```python
from build123d import *

# Parameters (mm, degrees)
F1_DEPTH     = 7.5
F2_R         = 1.5
F3_R         = 1.5
F4_F1_R      = 1
F4_F2_R      = 1
F5_W         = 10
F5_H         = 10
F6_DEPTH     = 1
F7_T1_DEPTH  = 5
F7_T3_DEPTH  = 7.5
F7_T9_DEPTH  = 11.0917464655
F7_T14_DEPTH = 15
F7_T22_DEPTH = 15
F7_T27_DEPTH = 11.0917464655


# Not quite as in the source:
# - a fillet or chamfer that OpenCascade refuses, or shapes differently, is made with other operations: its cross-section is extruded or revolved along the edge and cut away or added


with BuildPart() as f1:
    # F0 (on Front) → F1 (new body)
    with BuildSketch(Plane.XZ):
        Polygon((0, 0), (0, 5), (-14.5909318536, 5), (-495, 5), (-500, 5), (-500, 0), (-500, -195), (-495, -195), (-408.1860127931, -160.8005504943), align=None)
        Polygon((-26.1103633187, -4.911916504), (-410.018635385, -156.1485085302), (-495, -189.6260158027), (-495, -142.4539996661), (-495, -95.2819835295), (-495, -93.9333955313), (-494.06737982, -93.7563320577), align=None, mode=Mode.SUBTRACT)
        Polygon((-495, 0), (-27.044750547, 0), (-495, -88.8440800691), (-495, -44.4220400346), align=None, mode=Mode.SUBTRACT)
    extrude(amount=F1_DEPTH)

    # F2
    f2_edges = [f1.edges().sort_by_distance(p)[0] for p in [
        (-495, -3.75, -88.84408),
    ]]
    fillet(f2_edges, radius=F2_R)

    # F3
    f3_edges = [f1.edges().sort_by_distance(p)[0] for p in [
        (-495, -3.75, -93.933396),
        (-495, -3.75, 0),
        (-495, -3.75, -189.626016),
    ]]
    fillet(f3_edges, radius=F3_R)

    # F4: fillet of radius 1 on 2 edges, made by hand

    # F4_f1
    f4_f1_edges = [f1.edges().sort_by_distance(p)[0] for p in [
        (-27.044750547, -3.75, 0),
    ]]
    fillet(f4_f1_edges, radius=F4_F1_R)

    # F4_f2
    f4_f2_edges = [f1.edges().sort_by_distance(p)[0] for p in [
        (-26.1103633187, -3.75, -4.911916504),
    ]]
    fillet(f4_f2_edges, radius=F4_F2_R)

    # F5 (on face) → F6 (join)
    with BuildSketch(Plane.XY.offset(5)):
        with Locations((0, -3.75)):
            Rectangle(F5_W, F5_H)
    extrude(amount=F6_DEPTH)

    # F7: fillet of radius 3 on 3 edges, made by hand

    # F7_s2 → F7_t1 (join)
    with BuildSketch(Plane.YZ.offset(-5)):
        with BuildLine():
            ThreePointArc((-7.5, 2.5633014138), (-7.830730437, 3.9326078076), (-8.75, 5))
            Line((-8.75, 5), (-7.5, 5))
            Line((-7.5, 5), (-7.5, 2.5633014138))
        make_face()
        with BuildLine():
            ThreePointArc((1.25, 5), (0.330730437, 3.9326078076), (0, 2.5633014138))
            Line((0, 2.5633014138), (0, 5))
            Line((0, 5), (1.25, 5))
        make_face()
    extrude(amount=F7_T1_DEPTH)

    # F7_s4 → F7_t3 (join)
    with BuildSketch(Plane.XZ):
        with BuildLine():
            ThreePointArc((0, 2), (0.8786796564, 4.1213203436), (3, 5))
            Line((3, 5), (0, 5))
            Line((0, 5), (0, 2))
        make_face()
    extrude(amount=F7_T3_DEPTH)


with BuildPart() as f7_tool7:
    # F7_s8 → F7_t9 (new body)
    with BuildSketch(Plane.YZ.offset(-5)):
        with BuildLine():
            ThreePointArc((-7.5, 2.5633014138), (-7.830730437, 3.9326078076), (-8.75, 5))
            Line((-8.75, 5), (-7.5, 5))
            Line((-7.5, 5), (-7.5, 2.5633014138))
        make_face()
    extrude(amount=F7_T9_DEPTH)

    split(bisect_by=Plane.YZ, keep=Keep.TOP)

    split(bisect_by=Plane.YZ.offset(5), keep=Keep.BOTTOM)


with BuildPart() as f7_tool12:
    # F7_s13 → F7_t14 (new body)
    with BuildSketch(Plane.XZ):
        with BuildLine():
            ThreePointArc((0, 2), (0.8786796564, 4.1213203436), (3, 5))
            Line((3, 5), (0, 5))
            Line((0, 5), (0, 2))
        make_face()
    extrude(amount=F7_T14_DEPTH)

    split(bisect_by=Plane.XZ.offset(7.5), keep=Keep.TOP)

    split(bisect_by=Plane.XZ.offset(8.75), keep=Keep.BOTTOM)


with BuildPart() as f7_tool7_1:
    add(f7_tool7.part)

    # F7_t17: intersect F7_tool12
    add(f7_tool12.part, mode=Mode.INTERSECT)


with BuildPart() as f1_1:
    add(f1.part)

    # F7_t5: union F7_tool7
    add(f7_tool7_1.part)


with BuildPart() as f7_tool20:
    # F7_s21 → F7_t22 (new body)
    with BuildSketch(Plane.XZ.offset(-7.5)):
        with BuildLine():
            ThreePointArc((0, 2), (0.8786796564, 4.1213203436), (3, 5))
            Line((3, 5), (0, 5))
            Line((0, 5), (0, 2))
        make_face()
    extrude(amount=F7_T22_DEPTH)

    split(bisect_by=Plane.XZ, keep=Keep.BOTTOM)

    split(bisect_by=Plane.XZ.offset(-1.25), keep=Keep.TOP)


with BuildPart() as f7_tool25:
    # F7_s26 → F7_t27 (new body)
    with BuildSketch(Plane.YZ.offset(6.0917464655)):
        with BuildLine():
            ThreePointArc((1.25, 5), (0.330730437, 3.9326078076), (0, 2.5633014138))
            Line((0, 2.5633014138), (0, 5))
            Line((0, 5), (1.25, 5))
        make_face()
    extrude(amount=-F7_T27_DEPTH)

    split(bisect_by=Plane.YZ, keep=Keep.TOP)

    split(bisect_by=Plane.YZ.offset(5), keep=Keep.BOTTOM)


with BuildPart() as f7_tool20_1:
    add(f7_tool20.part)

    # F7_t30: intersect F7_tool25
    add(f7_tool25.part, mode=Mode.INTERSECT)


with BuildPart() as f1_2:
    add(f1_1.part)

    # F7_t18: union F7_tool20
    add(f7_tool20_1.part)


solid = f1_2.part
```
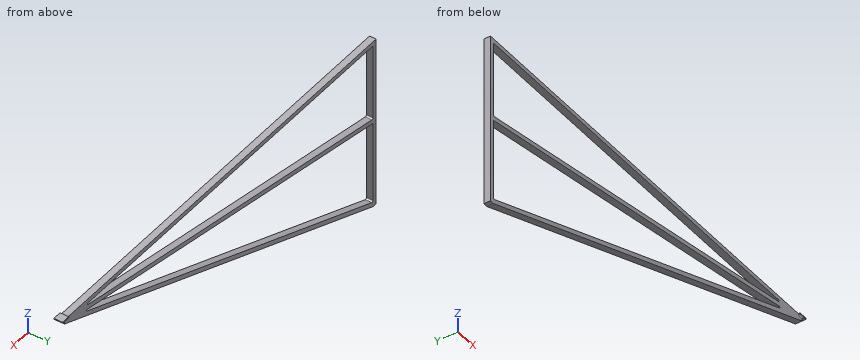
Geometry check sheet. Reference: the model listing, model coordinates, mm. Coordinates: 2 decimals unless noted, no trailing zeros. Write each loop counter-clockwise with the first axis right and the second up, starting at its lowest first coordinate (ties: lowest second). Pieces come first, ordered by that corner, then holes. Notation, with made-up numbers: M 3.5,20 L 21.5,20 A10 cw 21.5,29 Z; hole C -38,-19.75 d9. An arc over 180 degrees is marked long. Answer as a JSON object with one key per item and string values.
1. Section check B-B, the plane z = -136.5. Enter the section's corners in (x, y), plus the area to 3 significant figures.
Answers below:
{"outline": "M -500,-7.5 L -495,-7.5 L -495,0 L -500,0 Z; M -360.14,-7.5 L -346.5,-7.5 L -346.5,0 L -360.14,0 Z", "area": "140 mm²"}
2. Section check A-A, the plane x = -279. Enter the section's corners in (y, z), plus the area to 3 significant figures.
Answers below:
{"outline": "M -7.5,-109.91 L 0,-109.91 L 0,-104.54 L -7.5,-104.54 Z; M -7.5,-52.92 L 0,-52.92 L 0,-47.84 L -7.5,-47.84 Z; M -7.5,0 L 0,0 L 0,5 L -7.5,5 Z", "area": "116 mm²"}
3. Section check C-C, the plane z = -17.5. Enter the section's corners in (x, y).
Answers below:
{"outline": "M -500,-7.5 L -495,-7.5 L -495,0 L -500,0 Z; M -119.22,-7.5 L -92.41,-7.5 L -92.41,0 L -119.22,0 Z; M -58.06,-7.5 L -44.42,-7.5 L -44.42,0 L -58.06,0 Z"}
4. Scan lines: L1, parallel to Z at x = -292.5, y = -3.25; L2, parallel to Z at x = -327.5, y = -2; L3, parallel to Y at x = -284, z = -109.5. Record each from-to range of solid material in increasing order.
Answers below:
{"L1": "z = -115.23 to -109.85, -55.49 to -50.4, 0 to 5", "L2": "z = -129.02 to -123.64, -62.13 to -57.04, 0 to 5", "L3": "y = -7.5 to 0"}
5. Go/stop test with flat-tipped pins: pin 1 Ø1.5 at (x, y) = (-106.5, -2) entering from -Z; pin 2 Ø1.5 at (x, y) = (-344, -6) entering from -Z; pin 3 Ø4 at (x, y) = (-286.5, -5) entering from +Z. Record where each tip stops, or that it passes through.
Answers below:
{"pin 1": "stops at z = -42.25", "pin 2": "stops at z = -135.81", "pin 3": "stops at z = 5"}
6. Section check D-D, the plane y = -1.75. Give the number of separate pieces and of enclosed holes in the cut face, plus the area to 3 significant figures.
Answers below:
{"separate pieces": "1", "enclosed holes": "2", "area": "8,550 mm²"}
